```python
from build123d import *

# Parameters (mm, degrees)
EXTRUDE_1_DEPTH     = 40
FILLET_1_R          = 1.5
SKETCH_3_R          = 1.6
CUT_EXTRUDE_1_DEPTH = 40
SKETCH_4_R          = 2.1
CUT_EXTRUDE_2_DEPTH = 80
SKETCH_5_R          = 1.6
CUT_EXTRUDE_3_DEPTH = 80
CUT_EXTRUDE_4_DEPTH = 10
FILLET_4_R          = 1.5
EXTRUDE_2_DEPTH     = 1.5
FILLET_5_R          = 1.5
FILLET_6_R          = 1.5


with BuildPart() as part:
    # 草图2 → 凸台-拉伸1 (new body)
    with BuildSketch(Plane(origin=(0, 4.726404994, 0), x_dir=(1, 0, 0), z_dir=(0, 1, 0))):
        Polygon((21, 0), (-59, 0), (-59, -25), (-54, -25), (-54, -5), (16, -5), (16, -25), (21, -25), align=None)
    extrude(amount=-EXTRUDE_1_DEPTH)

    # 圆角1
    fillet_1_edges = [part.edges().sort_by_distance(p)[0] for p in [
        (16, -15.273595006, 5),
        (-54, -15.273595006, 5),
    ]]
    fillet(fillet_1_edges, radius=FILLET_1_R)

    # 草图3 → 切除-拉伸1 (cut)
    with BuildSketch(Plane.XY.offset(5)):
        with Locations((-22.5, -30.273595006)):
            Circle(SKETCH_3_R)
        with Locations((-22.5, -8.273595006)):
            Circle(SKETCH_3_R)
    extrude(amount=-CUT_EXTRUDE_1_DEPTH, mode=Mode.SUBTRACT)

    # 草图4 → 切除-拉伸2 (cut)
    with BuildSketch(Plane.ZY.offset(59)):
        with Locations(Location((17, -3.273595006, 0), (0, 0, 270))):
            Circle(SKETCH_4_R)
        with Locations(Location((17, -27.273595006, 0), (0, 0, 270))):
            Circle(SKETCH_4_R)
    extrude(amount=-CUT_EXTRUDE_2_DEPTH, mode=Mode.SUBTRACT)

    # 草图5 → 切除-拉伸3 (cut)
    with BuildSketch(Plane.XY.offset(5)):
        with Locations((-15.5, -30.273595006)):
            Circle(SKETCH_5_R)
        with Locations((-15.5, -11.773595006)):
            Circle(SKETCH_5_R)
    extrude(amount=-CUT_EXTRUDE_3_DEPTH, mode=Mode.SUBTRACT)

    # 草图7 → 切除-拉伸4 (cut)
    with BuildSketch(Plane.XY.offset(5)):
        with BuildLine():
            Line((-50.5, 4.726404994), (-42.933047922, -2.840547084))
            ThreePointArc((-42.933047922, -2.840547084), (-42.453382132, -3.161049518), (-41.887577755, -3.273595006))
            Line((-41.887577755, -3.273595006), (3.887577755, -3.273595006))
            ThreePointArc((3.887577755, -3.273595006), (4.453382132, -3.161049518), (4.933047922, -2.840547084))
            Line((4.933047922, -2.840547084), (12.5, 4.726404994))
            Line((12.5, 4.726404994), (-50.5, 4.726404994))
        make_face()
        with BuildLine():
            Line((12.5, -35.273595006), (-14.5, -35.273595006))
            Line((-14.5, -35.273595006), (-6.939339828, -27.712934835))
            ThreePointArc((-6.939339828, -27.712934835), (-6.452704805, -27.387775708), (-5.878679656, -27.273595006))
            Line((-5.878679656, -27.273595006), (3.887577755, -27.273595006))
            ThreePointArc((3.887577755, -27.273595006), (4.453382132, -27.386140495), (4.933047922, -27.706642929))
            Line((4.933047922, -27.706642929), (12.5, -35.273595006))
        make_face()
        with BuildLine():
            Line((-41.887577755, -27.273595006), (-32.121320344, -27.273595006))
            ThreePointArc((-32.121320344, -27.273595006), (-31.547295195, -27.387775708), (-31.060660172, -27.712934835))
            Line((-31.060660172, -27.712934835), (-23.5, -35.273595006))
            Line((-23.5, -35.273595006), (-50.5, -35.273595006))
            Line((-50.5, -35.273595006), (-42.933047922, -27.706642929))
            ThreePointArc((-42.933047922, -27.706642929), (-42.453382132, -27.386140495), (-41.887577755, -27.273595006))
        make_face()
    extrude(amount=-CUT_EXTRUDE_4_DEPTH, mode=Mode.SUBTRACT)

    # 圆角4
    fillet_4_edges = [part.edges().sort_by_distance(p)[0] for p in [
        (-50.5, 4.726404994, 2.5),
        (12.5, 4.726404994, 2.5),
        (-14.5, -35.273595006, 2.5),
        (12.5, -35.273595006, 2.5),
        (-50.5, -35.273595006, 2.5),
        (-23.5, -35.273595006, 2.5),
    ]]
    fillet(fillet_4_edges, radius=FILLET_4_R)

    # 草图6 → 凸台-拉伸2 (add, symmetric)
    with BuildSketch(Plane(origin=(0, -15.273595006, 0), x_dir=(-1, 0, 0), z_dir=(0, -1, 0))):
        Polygon((-16, -17), (9, -5), (-16, -5), align=None)
    extrude_2 = extrude(amount=EXTRUDE_2_DEPTH, both=True)

    # 圆角5
    fillet_5_edges = [part.edges().sort_by_distance(p)[0] for p in [
        (15.560660172, -16.773595006, 5.439339828),
        (15.560660172, -13.773595006, 5.439339828),
        (2.75, -13.773595006, 5),
        (2.75, -16.773595006, 5),
        (16, -16.773595006, 11.75),
        (16, -13.773595006, 11.75),
        (16, -15.273595006, 17),
        (-9, -15.273595006, 5),
    ]]
    fillet(fillet_5_edges, radius=FILLET_5_R)

    # 镜向2: 凸台-拉伸2 across plane
    add(extrude_2.mirror(Plane.ZY.offset(19)))

    # 圆角6
    fillet_6_edges = [part.edges().sort_by_distance(p)[0] for p in [
        (-53.560660172, -16.773595006, 5.439339828),
        (-53.560660172, -13.773595006, 5.439339828),
        (-40.75, -16.773595006, 5),
        (-29, -15.273595006, 5),
        (-54, -13.773595006, 11.75),
        (-40.75, -13.773595006, 5),
        (-54, -16.773595006, 11.75),
        (-54, -15.273595006, 17),
    ]]
    fillet(fillet_6_edges, radius=FILLET_6_R)


solid = part.part
```
CAD build for the part. Positions are in the model's coordinates, mm. A direction names the side the tool comes from. Give positions to 0.01 mm unless a question says otherwise; leave off trailing zeros. Order: outer loops, then holes, each group sorted by start corner. A loop starts at its lowest first (then second) coordinate and runs counter-clockwise, first axis right, second up. Notation, with made-up numbers: M 26,2.25 L 70,2.25 A23 ccw 70,40.25 Z; hole C 32.5,78 d4. An arc over 180 degrees is marked long. Put each result on its own line as item: value. Start each with the question number.
(1) Drill centre lines: line 1 along Y through (x, z) = (-22.5, 3.35); line 2 along Y through (x, z) = (18, 17.5); line 3 along X through (y, z) = (-23, 23.75). Where is each one in solid material? Low to high.
(2) Which spindle directions (+Z, -Z, +X, -X, +Y, -Y) get a long thin tool onto all of the face, cutting with end or side? Do faces 1 (the flat face through (-19, -3.274, 3)), 2 (the flat face through (-19, -15, 5)), 3 (the cylindrical face through (-53.549, -13.346, 12.142)), 4 (the flat face through (18, -15, 25)), 5 (the flat face through (-46.547, -31.32, 2.535)). Say none if no direction does.
(3) Saw through at A-A, the plane z = 22.5. Write the cut outline in (x, y), then the cut area to 3 significant figures.
(4) Flat gauge pins, fed straight in: pin 1 Ø8 at (x, z) = (4.5, 12) entering from +Y; pin 2 Ø4 at (x, z) = (-2.5, 3.5) entering from -Y; pin 3 Ø12 at (x, y) = (-17, -24.5) entering from +Z. Where does each tip first touch, or does it go through?
(5) Saw through at D-D, the plane z = 12.5. Write the cut outline in (x, y) (3 decimals), then the cut area to 3 significant figures.
(6) Saw through at B-B, the plane x = -38.5. Write the cut outline in (y, z), then the cut area to 3 significant figures.
(7) Saw through at C-C, the plane y = -23. Write the cut outline in (x, z), then the cut area to 3 significant figures.
(8) Mould opens along Y. For faces 6 (the flat face through (-10.55, -31.323, 2.535)), 7 (the flat face through (-18, -15, 0)), 8 (the cylindrical face through (-22.708, -28.687, 2.535)), 9 (the flat face through (-46.547, 0.773, 2.535)) say: +Y half, -Y half, draft (parallel to the pull), parting line (faces both ways), or undercut.
Check result:
1. line 1: y = -35.27 to -31.87, -28.67 to -9.87, -6.67 to -3.27
1. line 2: y = -35.27 to -29.31, -25.23 to -5.31, -1.23 to 4.73
1. line 3: x = -59 to -54, 16 to 21
2. face 1: +Z, -Z, +Y
2. face 2: +Z
2. face 3: +Z, +Y
2. face 4: +Z, +X, -X, +Y, -Y
2. face 5: +Z, -Z, -Y
3. outline: M -59,-35.27 L -54,-35.27 L -54,4.73 L -59,4.73 Z; M 16,-35.27 L 21,-35.27 L 21,4.73 L 16,4.73 Z
3. area: 400 mm2
4. pin 1: stops at y = -13.77
4. pin 2: stops at y = -27.27
4. pin 3: stops at z = 5
5. outline: M -59,-35.274 L -54,-35.274 L -54,-18.274 A1.5 cw -52.5,-16.774 L -44.625,-16.774 L -44.625,-13.774 L -52.5,-13.774 A1.5 cw -54,-12.274 L -54,4.726 L -59,4.726 Z; M 6.625,-16.774 L 14.5,-16.774 A1.5 cw 16,-18.274 L 16,-35.274 L 21,-35.274 L 21,4.726 L 16,4.726 L 16,-12.274 A1.5 cw 14.5,-13.774 L 6.625,-13.774 Z
5. area: 458 mm2
6. outline: M -27.27,0 L -3.27,0 L -3.27,5 L -12.27,5 A1.5 cw -13.77,6.5 L -13.77,9.56 L -16.77,9.56 L -16.77,6.5 A1.5 cw -18.27,5 L -27.27,5 Z
6. area: 135 mm2
7. outline: M -59,0 L 21,0 L 21,25 L 16,25 L 16,6.5 A1.5 cw 14.5,5 L -52.5,5 A1.5 cw -54,6.5 L -54,25 L -59,25 Z
7. area: 601 mm2
8. face 6: -Y half
8. face 7: draft
8. face 8: undercut
8. face 9: +Y half
